Read the model definition and answer for the solid it produces. Units are mm, in the model's axes. A direction names the side the tool comes from. Round coordinates to 2 decimals unless told otherwise and drop trailing zeros. Loops run counter-clockwise (first coordinate to the right, second up) from the corner with the lowest first, then second, coordinate; pieces in that order, holes last. Notation, with made-up numbers: (11, -15.75) - (58, -15.75) arc R27 ccw to (58, 11.25) - close; hole circle Ø4 at (11, 82.5). An arc over 180 degrees is marked (long way). Use CSV: the item, a comma, the result in double quotes. Start each with the question number.
1. Find section B-B (y = 3.5). Give the vertices of the cut face in (x, z).
2. Find section C-C (y = 11). Give the vertices of the cut face in (x, z).
3. Consider line 1 along Y through (x, z) = (2.25, -2.25); line 2 along X through (y, z) = (10, -1.5); line 3 along Y through (x, z) = (-0.75, -0.75). Determine where each line is inside the solid, lowest interval first.
4. A tool of negligible diameter and unlimited length cuts with its end or side. For faces 1 (the cylindrical face through (-0.434, 17.246, 1.952)), 2 (the flat face through (1.08, 20.52, 0.63)), 3 (the flat face through (-1, 8, -2)), 4 (the flat face through (-2, 22, 0)), 5 (the flat face through (0, 0, 0)), from which of +Z, -Z, +X, -X, +Y, -Y can it reach the whole face along a straight path? Write none if from no direction.
5. Determine the mould class of faces 6 (the flat face through (-1.08, 20.52, -0.63)), 7 (the cylindrical face through (-0.59, 19.73, -4.46)), 8 (the flat face through (2, 18, 2)) for opening direction X: +X half, -X half, draft (parallel to the pull), parting line (faces both ways), or undercut.
6. Given pin 1 Ø3 at (x, z) = (0.5, 0) entering from +Y; pin 2 Ø5 at (x, y) = (1, 6) entering from -Z, each flat-ended and moving along its own axis, determine where each tip first touches the part or whether it passes through.
from build123d import *

# Parameters (mm, degrees)
CUT_EXTRUDE1_DEPTH = 3


with BuildPart() as part:
    # Sketch1 → Revolve1 (revolve)
    with BuildSketch(Plane.XY):
        with BuildLine():
            Line((0, 0), (0, 22))
            Line((0, 22), (4, 22))
            Line((4, 22), (4.5, 21.5))
            Line((4.5, 21.5), (4.5, 18))
            Line((4.5, 18), (2.5, 18))
            ThreePointArc((2.5, 18), (2.146446609, 17.853553391), (2, 17.5))
            Line((2, 17.5), (2, 17))
            Line((2, 17), (2.5, 16.5))
            Line((2.5, 16.5), (2.5, 8))
            Line((2.5, 8), (2, 8))
            ThreePointArc((2, 8), (1.505025253, 7.794974747), (1.3, 7.3))
            Line((1.3, 7.3), (1.3, 6.7))
            Line((1.3, 6.7), (2, 6))
            Line((2, 6), (2, 0.7))
            Line((2, 0.7), (1.3, 0))
            Line((1.3, 0), (0, 0))
        make_face()
    revolve(axis=Axis((0, 0, 0), (0, 1, 0)))

    # Sketch2 → Cut-Extrude1 (cut)
    with BuildSketch(Plane(origin=(0, 22, 0), x_dir=(1, 0, 0), z_dir=(0, 1, 0))):
        Polygon((0.721687836, 1.25), (-0.721687836, 1.25), (-1.443375673, 0), (-0.721687836, -1.25), (0.721687836, -1.25), (1.443375673, 0), align=None)
    extrude(amount=-CUT_EXTRUDE1_DEPTH, mode=Mode.SUBTRACT)


solid = part.part
Filled sheet:
1,outline,"circle Ø4 at (0, 0)"
2,outline,"circle Ø5 at (0, 0)"
3,line 1,"y = 18 to 22"
3,line 2,"x = -2 to 2"
3,line 3,"y = 0 to 19"
4,face 1,"none"
4,face 2,"+Y"
4,face 3,"-Y"
4,face 4,"+Z, -Z, +X, -X, +Y"
4,face 5,"+Z, -Z, +X, -X, -Y"
5,face 6,"undercut"
5,face 7,"parting line"
5,face 8,"draft"
6,pin 1,"stops at y = 22"
6,pin 2,"stops at z = -2.5"
